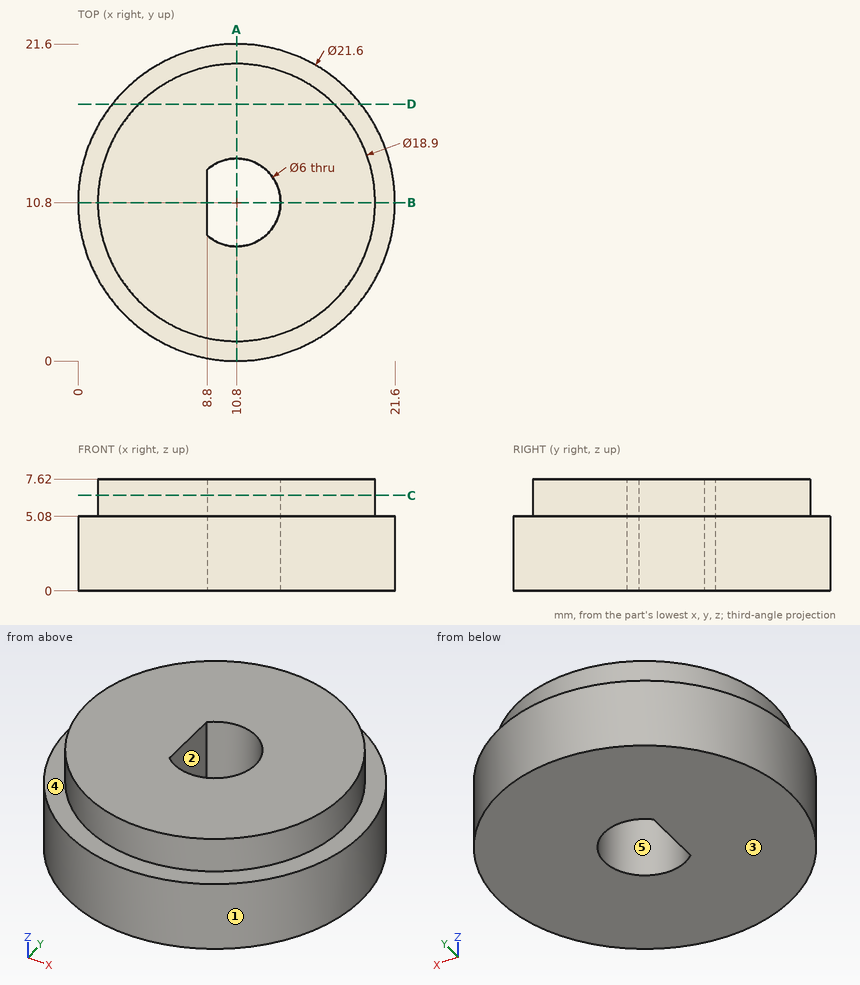
Here's the drawing with two shaded views (mm, measured from the low corner). I have some questions. A direction names the side the tool comes from. Round coordinates to 2 decimals unless told otherwise and drop trailing zeros. Loops run counter-clockwise (first coordinate to the right, second up) from the corner with the lowest first, then second, coordinate; pieces in that order, holes last. Notation, with made-up numbers: (0, -31.75) -> (48, -31.75) arc R20 ccw to (48, -24.75) -> close; hole circle Ø9 at (-11, -3.75). An arc over 180 degrees is marked (long way). Answer as CSV lines item,"result". Start each with the question number.
1. For the marked faces 4 and 5, which set-ups out of +Z, -Z, +X, -X, +Y, -Y let a thin tool reach every point of the face, with its end or its side?
2. I need wall thicknesses on probe 1 along Y at (x, z) = (10.8, 5); probe 2 along Y at (x, z) = (10.8, 5.5); probe 3 along Z at (x, y) = (16.25, 2). Which ranges of each line are inside material? Lowest first, please. Write a range as from..to.
3. Imagine slicing it at A-A on x = 10.8. Write out the boundary of the cut face in (y, z).
4. If we mould it in two halves opening along Y, with no side actions, what happens to the marked faces 1, 2 and 3? For each: pulls with the +Y half, pulls with the -Y half, needs draft (parallel to the pull), parting line crosses it, or undercut.
5. I'm going to push a flat-ended pin straight in: P1, Ø1.3, axis at y = 10, z = 2.5, coming from the +X side. Where does the tip first touch, or does it pass through?
6. Imagine slicing it at C-C on z = 6.5. Write out the boundary of the cut face in (x, y), plus the area to 3 significant figures.
7. Imagine slicing it at B-B on y = 10.8. Write out the boundary of the cut face in (x, z), plus the area to 3 significant figures.
8. Imagine slicing it at D-D on y = 17.5. Write out the boundary of the cut face in (x, z).
Solution:
1,face 4,"+Z"
1,face 5,"+Z, -Z"
2,probe 1,"0..7.8, 13.8..21.6"
2,probe 2,"1.35..7.8, 13.8..20.25"
2,probe 3,"0..5.08"
3,outline,"(0, 0) -> (7.8, 0) -> (7.8, 7.62) -> (1.35, 7.62) -> (1.35, 5.08) -> (0, 5.08) -> close; (13.8, 0) -> (21.6, 0) -> (21.6, 5.08) -> (20.25, 5.08) -> (20.25, 7.62) -> (13.8, 7.62) -> close"
4,face 1,"parting line crosses it"
4,face 2,"undercut"
4,face 3,"needs draft"
5,P1,"x = 21.6"
6,outline,"circle Ø18.9 at (10.8, 10.8); hole (8.8, 8.56) arc R3 ccw (long way) to (8.8, 13.04) -> close"
6,area,"255 mm²"
7,outline,"(0, 0) -> (8.8, 0) -> (8.8, 7.62) -> (1.35, 7.62) -> (1.35, 5.08) -> (0, 5.08) -> close; (13.8, 0) -> (21.6, 0) -> (21.6, 5.08) -> (20.25, 5.08) -> (20.25, 7.62) -> (13.8, 7.62) -> close"
7,area,"120 mm²"
8,outline,"(2.33, 0) -> (19.27, 0) -> (19.27, 5.08) -> (17.46, 5.08) -> (17.46, 7.62) -> (4.14, 7.62) -> (4.14, 5.08) -> (2.33, 5.08) -> close"
